Part model, mm, in its own coordinate system. Face numbers are marked on the shaded views. A direction names the side the tool comes from. Give positions to 0.01 mm unless a question says otherwise; leave off trailing zeros. Write each loop counter-clockwise with the first axis right and the second up, starting at its lowest first coordinate (ties: lowest second). Pieces come first, ordered by that corner, then holes. Notation, with made-up numbers: M 77.5,40.25 L 130.5,40.25 A21 cw 130.5,55.25 Z; hole C -37,88.25 d1. An arc over 180 degrees is marked long. Use a Markdown table: item, result.
```python
from build123d import *

# Parameters (mm, degrees)
SKETCH_1_R          = 1.5
EXTRUDE_1_DEPTH     = 5
EXTRUDE_2_DEPTH     = 30
SKETCH_3_R          = 1.5
CUT_EXTRUDE_1_DEPTH = 5


with BuildPart() as part:
    # 草图1 → 凸台-拉伸1 (new body)
    with BuildSketch(Plane(origin=(0, 0, 0), x_dir=(1, 0, 0), z_dir=(0, 1, 0))):
        Circle(SKETCH_1_R)
    extrude(amount=EXTRUDE_1_DEPTH)

    # 草图2 → 凸台-拉伸2 (add)
    with BuildSketch(Plane(origin=(0, 5, 0), x_dir=(1, 0, 0), z_dir=(0, 1, 0))):
        Polygon((0, 2.309401077), (-2, 1.154700538), (-2, -1.154700538), (0, -2.309401077), (2, -1.154700538), (2, 1.154700538), align=None)
    extrude(amount=EXTRUDE_2_DEPTH)

    # 草图3 → 切除-拉伸1 (cut)
    with BuildSketch(Plane(origin=(0, 35, 0), x_dir=(1, 0, 0), z_dir=(0, 1, 0))):
        Circle(SKETCH_3_R)
    extrude(amount=-CUT_EXTRUDE_1_DEPTH, mode=Mode.SUBTRACT)


solid = part.part
```
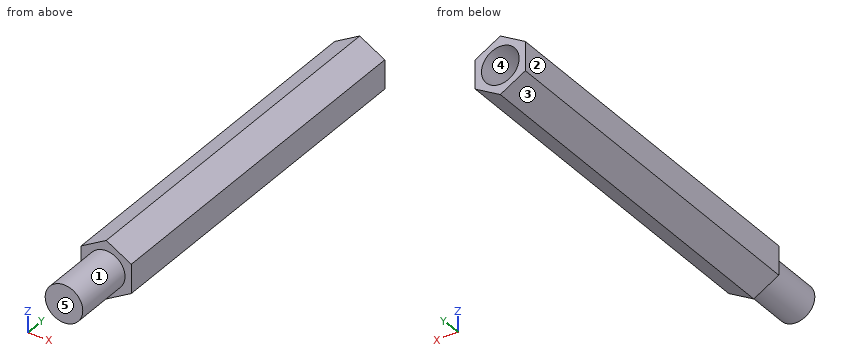
1. Cut at B-B, the plane z = 0. Give the cut face in (x, y).
Findings below:
| item | result |
|---|---|
| outline | M -2,5 L -1.5,5 L -1.5,0 L 1.5,0 L 1.5,5 L 2,5 L 2,35 L 1.5,35 L 1.5,30 L -1.5,30 L -1.5,35 L -2,35 Z |
2. Drill centre lines: L1, parallel to X at y = 33.85, z = 0; L2, parallel to Y at x = 1.15, z = -1.3; L3, parallel to Y at x = 0.4, z = 1. Where is each one in solid material? Low to high.
Findings below:
| item | result |
|---|---|
| L1 | -2 to -1.5, 1.5 to 2 |
| L2 | 5 to 35 |
| L3 | 0 to 30 |
3. Tool access for the marked faces 1 and 2: list every direction of +Z, -Z, +X, -X, +Y, -Y with a clear straight run to the whole face (end or side of a thin tool).
Findings below:
| item | result |
|---|---|
| face 1 | -Y |
| face 2 | +Z, -Z, -X, +Y, -Y |
4. Cut at D-D, the plane y = 10. Give the cut face in (x, z).
Findings below:
| item | result |
|---|---|
| outline | M -2,-1.15 L 0,-2.31 L 2,-1.15 L 2,1.15 L 0,2.31 L -2,1.15 Z |
5. Cut at C-C, the plane x = 0.9. Give the cut face in (y, z), then the cut area to 3 significant figures.
Findings below:
| item | result |
|---|---|
| outline | M 0,-1.2 L 5,-1.2 L 5,-1.79 L 35,-1.79 L 35,-1.2 L 30,-1.2 L 30,1.2 L 35,1.2 L 35,1.79 L 5,1.79 L 5,1.2 L 0,1.2 Z |
| area | 107 mm2 |
6. Drop flat-ended pins along their axis: P1, Ø2, axis at x = 0.5, y = 20.5, coming from the +Z side; P2, Ø0.9, axis at x = -0.5, z = 0, coming from the +Y side; P3, Ø1, axis at x = -1.5, y = 5, coming from the +Z side. Give the stop position or say it passes through.
Findings below:
| item | result |
|---|---|
| P1 | z = 2.31 |
| P2 | y = 30 |
| P3 | z = 1.73 |
7. Two-plate mould, pull along Z, no slides. Class the marked faces 3, 4 and 5: released by +Z, released by -Z, zero draft, split by the parting line, or undercut.
Findings below:
| item | result |
|---|---|
| face 3 | released by -Z |
| face 4 | undercut |
| face 5 | zero draft |
8. Cut at A-A, the plane y = 31. Give the cut face in (x, z).
Findings below:
| item | result |
|---|---|
| outline | M -2,-1.15 L 0,-2.31 L 2,-1.15 L 2,1.15 L 0,2.31 L -2,1.15 Z; hole C 0,0 d3 |
